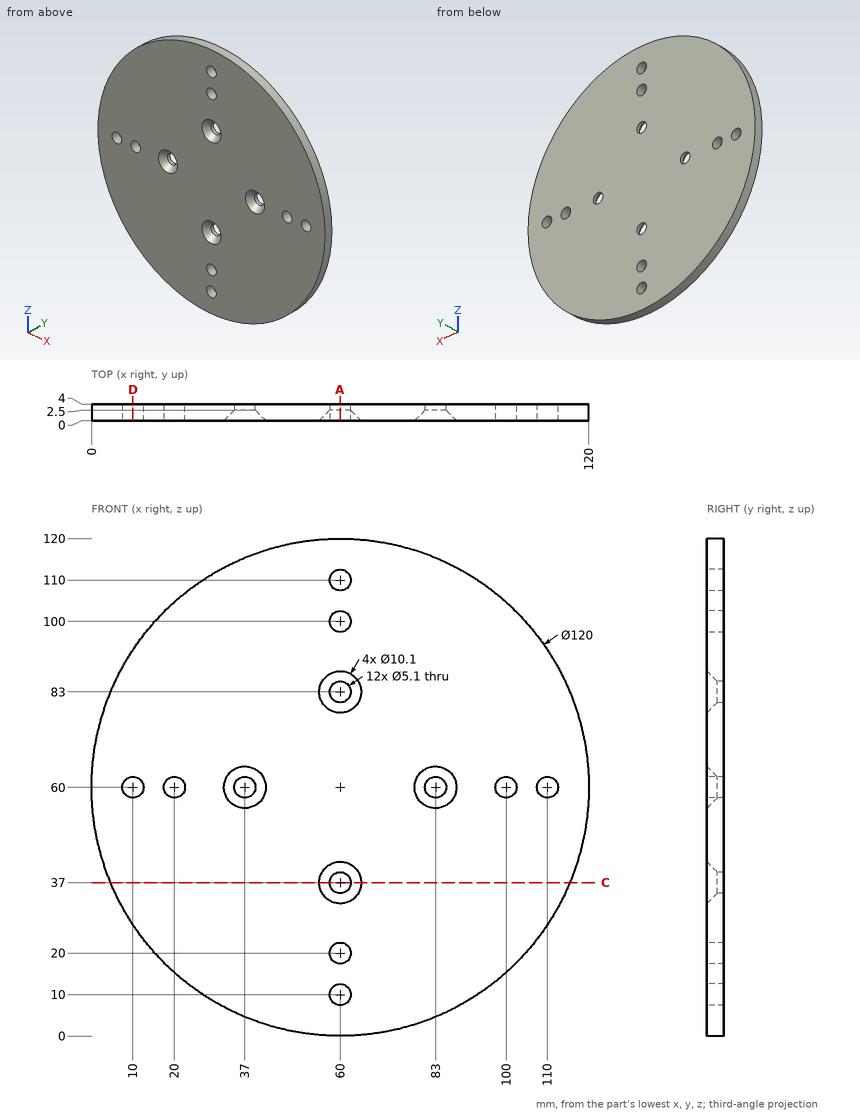
Here's the drawing with two shaded views (mm, measured from the low corner). I have some questions. Round coordinates to 2 decimals unless told otherwise and drop trailing zeros. Loops run counter-clockwise (first coordinate to the right, second up) from the corner with the lowest first, then second, coordinate; pieces in that order, holes last.
1. Will these pins go through, and if not, where does the flat tip stop? pin 1 (1.5 mm diameter, centred on x = 72.5, y = 0.5, fed in from +Z); pin 2 (8 mm diameter, centred on x = 60, z = 37, fed in from -Y); pin 3 (1 mm diameter, centred on x = 94, y = 3, fed in from -Z).
Answers:
pin 1: stops at z = 118.84
pin 2: stops at y = 1.05
pin 3: stops at z = 10.22
2. Suppose I cut it at A-A, the plane x = 60. Give the number of separate pieces and of enclosed holes in the cut face, and give its area (3 significant figures).
Answers:
separate pieces: 7
enclosed holes: 0
area: 345 mm2
3. Suppose I cut it at C-C, the plane z = 37. Please give me the cut outline in (x, y), and give its area (3 significant figures).
Answers:
outline: (4.58, 0) - (54.95, 0) - (57.45, 2.5) - (57.45, 4) - (4.58, 4) - close; (62.55, 2.5) - (65.05, 0) - (115.42, 0) - (115.42, 4) - (62.55, 4) - close
area: 417 mm2
4. If I drill on probe 1 along Z at (x, y) = (100, 3.1); probe 2 along Z at (x, y) = (110, 2.45), over which ranges is the centre line in solid material (lowest first)?
Answers:
probe 1: z = 15.28 to 57.45, 62.55 to 104.72
probe 2: z = 26.83 to 57.45, 62.55 to 93.17
5. Suppose I cut it at D-D, the plane x = 10. Please give me the cut outline in (y, z).
Answers:
outline: (0, 26.83) - (4, 26.83) - (4, 57.45) - (0, 57.45) - close; (0, 62.55) - (4, 62.55) - (4, 93.17) - (0, 93.17) - close
